Autodesk Inventor part; units mm, degrees
ref_plane "YZ Plane" through (0, 0, 0) normal (1, 0, 0) x (0, 1, 0)
ref_plane "XZ Plane" through (0, 0, 0) normal (0, 1, 0) x (-1, 0, 0)
sketch "Sketch1" plane through (0, 0, 0) normal (0, 0, 1) x (1, 0, 0)
  circle A0 centre (0, 0) radius 37.465
  dimension "d0" = 74.93
extrude "Extrusion1" add sketch "Sketch1" along normal blind 25.4
sketch "Sketch3" plane through (0, 0, 25.4) normal (0, 0, 1) x (1, 0, 0)
  circle A0 centre (0, 0) radius 26.289
  dimension "d6" = 52.578
extrude "Extrusion3" cut sketch "Sketch3" against normal blind 2.54
sketch "Sketch4" plane through (0, 0, 0) normal (0, 0, -1) x (-1, 0, 0)
  circle A0 centre (0, 0) radius 26.289
  dimension "d9" = 52.578
extrude "Extrusion4" cut sketch "Sketch4" against normal blind 2.54
ref_plane "Work Plane1" through (0, 0, 12.7) normal (0, 0, 1) x (1, 0, 0)
sketch "Sketch5" plane through (0, 0, 12.7) normal (0, 0, 1) x (1, 0, 0)
  circle A0 centre (0, 0) radius 29.337
  circle A1 centre (0, 0) radius 37.465
  dimension "d13" = 58.674
  dimension "d34" = 74.93
extrude "Extrusion5" cut sketch "Sketch5" along normal mid plane 19.304
ref_plane "Work Plane2" through (0, 0, 20.1676) normal (0, 0, 1) x (1, 0, 0)
sketch "Sketch6" plane through (0, 0, 20.1676) normal (0, 0, 1) x (1, 0, 0)
  circle A0 centre (0, 0) radius 29.337
  dimension "d17" = 58.674
loft "Loft1" add profiles "Sketch6" section 1 edges at (-37.465, 0, 22.352)
ref_plane "Work Plane3" through (0, 0, 5.2324) normal (0, 0, 1) x (1, 0, 0)
sketch "Sketch7" plane through (0, 0, 5.2324) normal (0, 0, 1) x (1, 0, 0)
  circle A0 centre (0, 0) radius 29.337
  dimension "d31" = 58.674
loft "Loft3" add profiles "Sketch7" section 1 edges at (-37.465, 0, 3.048)
sketch "Sketch2" plane through (0, 0, 25.4) normal (0, 0, 1) x (1, 0, 0)
  circle A0 centre (0, 0) radius 26.289
  dimension "d3" = 52.578
extrude "Extrusion2" cut sketch "Sketch2" against normal blind 50.8
ref_plane "Work Plane4" through (0, 0, 22.352) normal (0, 0, 1) x (1, 0, 0)
ref_plane "Work Plane5" through (0, 0, 3.048) normal (0, 0, 1) x (1, 0, 0)
properties part number "KF50tube_v2"
Model file for the job. Use its own axes, mm. A direction names the side the tool comes from. Give positions to 0.01 mm unless a question says otherwise; leave off trailing zeros. Loops run counter-clockwise (first coordinate to the right, second up) from the corner with the lowest first, then second, coordinate; pieces in that order, holes last.
Item 1: Slice it at A-A (x = 0). Write the cut outline in (y, z) (3 decimals), plus the area to 3 significant figures.
Check values:
outline: (-37.465, 0) - (-26.289, 0) - (-26.289, 25.4) - (-37.465, 25.4) - (-37.465, 22.352) - (-29.337, 20.168) - (-29.337, 5.232) - (-37.465, 3.048) - close; (26.289, 0) - (37.465, 0) - (37.465, 3.048) - (29.337, 5.232) - (29.337, 20.168) - (37.465, 22.352) - (37.465, 25.4) - (26.289, 25.4) - close
area: 289 mm2
Item 2: Slice it at B-B (z = 14.25). Write the cut outline in (x, y), plus the area to 3 significant figures.
Check values:
outline: circle Ø58.67 at (0, 0); hole circle Ø52.58 at (0, 0)
area: 533 mm2
Item 3: Mould opens along Z. For faces 3 (the face through (-21.62, 19.83, 12.8)), 4 (the face through (-26, -8, 0)), 5 (the face through (-29.73, 22.8, 23.85)), 6 (the face through (-26, -8, 25.4)) say: +Z half, -Z half, draft (parallel to the pull), parting line (faces both ways), or undercut.
Check values:
face 3: undercut
face 4: -Z half
face 5: draft
face 6: +Z half
Item 4: Drill centre lines: line 1 along Y through (x, z) = (0, 6); line 2 along X through (y, z) = (-1.5, 23.25); line 3 along Y through (x, z) = (17, 10.75). Where is each one in solid material? Low to high.
Check values:
line 1: y = -29.34 to -26.29, 26.29 to 29.34
line 2: x = -37.43 to -26.25, 26.25 to 37.43
line 3: y = -23.91 to -20.05, 20.05 to 23.91
Item 5: Drop flat-ended pins along their axis: P1, Ø8, axis at x = 16, y = -16.5, coming from the +Z side; P2, Ø10, axis at x = 27.5, z = 12, coming from the -Y side; P3, Ø2, axis at x = 15.5, z = 15, coming from the +Y side; P4, Ø6, axis at x = 10.5, z = 11, coming from the +Y side. Give the stop position or say it passes through.
Check values:
P1: stops at z = 25.4
P2: stops at y = -18.83
P3: stops at y = 25.5
P4: stops at y = 28.36
Item 6: Which spindle directions (+Z, -Z, +X, -X, +Y, -Y) get a long thin tool onto all of the face, cutting with end or side? Do faces 1 (the face through (-3.885, 29.591, 20.304)), 2 (the face through (-29.73, 22.8, 1.5)). Say none if no direction does.
Check values:
face 1: none
face 2: +Z, -Z
